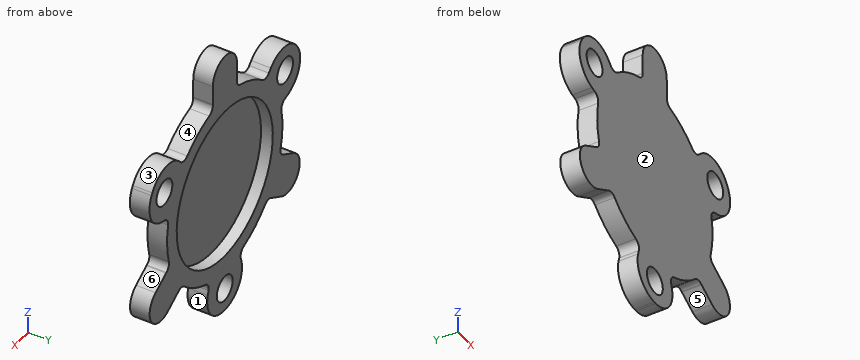
```python
from build123d import *

# Parameters (mm, degrees)
SKETCH1_R           = 20
BOSS_EXTRUDE1_DEPTH = 2
SKETCH2_R           = 35
SKETCH2_R_2         = 20
SKETCH2_R_3         = 3.3
BOSS_EXTRUDE2_DEPTH = 5
CUT_EXTRUDE1_DEPTH  = 10
FILLET1_R           = 2
FILLET2_R           = 7
BOSS_EXTRUDE3_DEPTH = 5
FILLET3_R           = 2


with BuildPart() as part:
    # Sketch1 → Boss-Extrude1 (new body)
    with BuildSketch(Plane(origin=(0, 0, 0), x_dir=(1, 0, 0), z_dir=(0, 1, 0))):
        with Locations(Location((0, 0, 0), (0, 0, 270))):
            Circle(SKETCH1_R)
    extrude(amount=BOSS_EXTRUDE1_DEPTH)

    # Sketch2 → Boss-Extrude2 (add)
    with BuildSketch(Plane(origin=(0, 0, 0), x_dir=(1, 0, 0), z_dir=(0, 1, 0))):
        with Locations(Location((0, 0, 0), (0, 0, 270))):
            Circle(SKETCH2_R)
        with Locations(Location((0, 0, 0), (0, 0, 270))):
            Circle(SKETCH2_R_2, mode=Mode.SUBTRACT)
        with Locations(Location((0, 29, 0), (0, 0, 270))):
            Circle(SKETCH2_R_3, mode=Mode.SUBTRACT)
        with Locations(Location((25.11473671, -14.5, 0), (0, 0, 270))):
            Circle(SKETCH2_R_3, mode=Mode.SUBTRACT)
        with Locations(Location((-25.11473671, -14.5, 0), (0, 0, 270))):
            Circle(SKETCH2_R_3, mode=Mode.SUBTRACT)
    extrude(amount=BOSS_EXTRUDE2_DEPTH)

    # Sketch3 → Cut-Extrude1 (cut)
    with BuildSketch(Plane(origin=(0, 5, 0), x_dir=(1, 0, 0), z_dir=(0, 1, 0))):
        with BuildLine():
            ThreePointArc((-23.193270109, -6.170269172), (-20.763157745, 12.037079399), (-6.170269172, 23.193270109))
            Line((-6.170269172, 23.193270109), (-14.951119735, 56.199389167))
            Line((-14.951119735, 56.199389167), (-49.377364183, -13.136208329))
            Line((-49.377364183, -13.136208329), (-23.193270109, -6.170269172))
        make_face()
        with BuildLine():
            Line((13.312391969, 49.330155919), (6.253025204, 23.171095697))
            ThreePointArc((6.253025204, 23.171095697), (20.805995419, 11.96288237), (23.171095697, -6.253025204))
            Line((23.171095697, -6.253025204), (56.145658563, -15.151645078))
            Line((56.145658563, -15.151645078), (13.312391969, 49.330155919))
        make_face()
        with BuildLine():
            Line((36.064972214, -36.193947589), (16.940244905, -17.000826525))
            ThreePointArc((16.940244905, -17.000826525), (-0.042837674, -23.999961769), (-17.000826525, -16.940244905))
            Line((-17.000826525, -16.940244905), (-41.194538828, -41.047744089))
            Line((-41.194538828, -41.047744089), (36.064972214, -36.193947589))
        make_face()
    extrude(amount=-CUT_EXTRUDE1_DEPTH, mode=Mode.SUBTRACT)

    # Fillet1
    fillet1_edges = [part.edges().sort_by_distance(p)[0] for p in [
        (16.940244905, 2.5, 17.000826525),
        (-17.000826525, 2.5, 16.940244905),
        (6.253025204, 2.5, -23.171095697),
        (23.171095697, 2.5, 6.253025204),
        (-6.170269172, 2.5, -23.193270109),
        (-23.193270109, 2.5, 6.170269172),
    ]]
    fillet(fillet1_edges, radius=FILLET1_R)

    # Fillet2
    fillet2_edges = [part.edges().sort_by_distance(p)[0] for p in [
        (-24.792872016, 2.5, 24.70452382),
        (24.70452382, 2.5, 24.792872016),
        (33.791181225, 2.5, 9.118995089),
        (9.118995089, 2.5, -33.791181225),
        (-8.998309209, 2.5, -33.823518909),
        (-33.823518909, 2.5, 8.998309209),
    ]]
    fillet(fillet2_edges, radius=FILLET2_R)

    # Sketch4 → Boss-Extrude3 (add)
    with BuildSketch(Plane(origin=(0, 5, 0), x_dir=(1, 0, 0), z_dir=(0, 1, 0))):
        with BuildLine():
            Line((-23.70496499, 19.52200868), (-19.379307126, 17.014283806))
            ThreePointArc((-19.379307126, 17.014283806), (-17.561374138, 10.180901067), (-24.394756876, 8.362968079))
            Line((-24.394756876, 8.362968079), (-28.720414739, 10.870692953))
            ThreePointArc((-28.720414739, 10.870692953), (-30.538347728, 17.704075692), (-23.70496499, 19.52200868))
        make_face()
        with BuildLine():
            Line((23.774503624, 19.437262295), (19.439921245, 16.944995134))
            ThreePointArc((19.439921245, 16.944995134), (17.597606027, 10.118145595), (24.424455566, 8.275830376))
            Line((24.424455566, 8.275830376), (28.759037945, 10.768097537))
            ThreePointArc((28.759037945, 10.768097537), (30.601353164, 17.594947076), (23.774503624, 19.437262295))
        make_face()
        with BuildLine():
            Line((4.945911115, -30.307955248), (4.954835631, -25.307963213))
            ThreePointArc((4.954835631, -25.307963213), (-0.036231889, -20.299046662), (-5.04514844, -25.290114182))
            Line((-5.04514844, -25.290114182), (-5.054072955, -30.290106217))
            ThreePointArc((-5.054072955, -30.290106217), (-0.063005435, -35.299022768), (4.945911115, -30.307955248))
        make_face()
    extrude(amount=-BOSS_EXTRUDE3_DEPTH)

    # Fillet3
    fillet3_edges = [part.edges().sort_by_distance(p)[0] for p in [
        (-18.017295098, 2.5, -15.854875507),
        (-22.711825842, 2.5, -7.757123623),
        (22.739372512, 2.5, -7.675997509),
        (18.073779039, 2.5, -15.790456334),
        (-4.722077413, 2.5, 23.530873016),
        (4.638046803, 2.5, 23.547579957),
    ]]
    fillet(fillet3_edges, radius=FILLET3_R)


solid = part.part
```
Build history of the part. All positions in model axes, mm. Face numbers are marked on the shaded views. A direction names the side the tool comes from. Round coordinates to 2 decimals unless told otherwise and drop trailing zeros. Write each loop counter-clockwise with the first axis right and the second up, starting at its lowest first coordinate (ties: lowest second). Pieces come first, ordered by that corner, then holes. Notation, with made-up numbers: (33.5, 31) - (73.5, 31) arc R24 cw to (73.5, 42) - close; hole circle Ø6 at (4.5, -29.75). An arc over 180 degrees is marked (long way). Answer as CSV lines item,"result".
Q1. Cut at D-D (y = 1.05). State how many separate pieces and enclosed holes the cut face has, and give its area (3 significant figures).
Report:
separate pieces,"1"
enclosed holes,"3"
area,"2,440 mm^2"
Q2. Pull direction X, two halves, no side cores. Call the marked faces 1, 2 and 3: +X half, -X half, draft (parallel to the pull), parting line (faces both ways), or undercut.
Report:
face 1,"+X half"
face 2,"draft"
face 3,"undercut"
Q3. Tool access for the marked faces 4, 5 and 6: list every direction of +Z, -Z, +X, -X, +Y, -Y with a clear straight run to the whole face (end or side of a thin tool).
Report:
face 4,"+Z, +Y, -Y"
face 5,"-Z, +Y, -Y"
face 6,"+X, +Y, -Y"
Q4. Cut at A-A (z = 14.5). Write the cut outline in (x, y).
Report:
outline,"(-31.36, 0) - (-28.41, 0) - (-28.41, 5) - (-31.36, 5) - close; (-21.81, 0) - (21.81, 0) - (21.81, 5) - (13.77, 5) - (13.77, 2) - (-13.77, 2) - (-13.77, 5) - (-21.81, 5) - close; (28.41, 0) - (31.32, 0) - (31.32, 5) - (28.41, 5) - close"
Q5. Drill centre lines: probe 1 along Z at (x, y) = (-26, 3.2); probe 2 along X at (y, z) = (3.55, 12.5); probe 3 along X at (y, z) = (1.8, 14.5). Where is each one in solid material? Low to high. Write a range as [from, to].
Report:
probe 1,"z = [-20.19, -9.29], [6.92, 11.32], [17.68, 20.93]"
probe 2,"x = [-31.29, -27.74], [-22.49, -15.61], [15.61, 22.49], [27.74, 31.22]"
probe 3,"x = [-31.36, -28.41], [-21.81, 21.81], [28.41, 31.32]"
Q6. Cut at C-C (z = -29). Write the cut outline in (x, y), and give its area (3 significant figures).
Report:
outline,"(-7.13, 0) - (-3.3, 0) - (-3.3, 5) - (-7.13, 5) - close; (3.3, 0) - (7.23, 0) - (7.23, 5) - (3.3, 5) - close"
area,"38.8 mm^2"
Q7. Drop flat-ended pins along their axis: pin 1 (6 mm diameter, centred on x = 13, z = -24, fed in from +Y); pin 2 (2 mm diameter, centred on x = 20.5, y = 0.5, fed in from -Z); pin 3 (12 mm diameter, centred on x = -8.5, z = -9.5, fed in from +Y). Give the stop position or say it passes through.
Report:
pin 1,"passes through"
pin 2,"stops at z = -18.13"
pin 3,"stops at y = 2"
Q8. Cut at B-B (z = 0). Write the cut outline in (x, y).
Report:
outline,"(-24, 0) - (24, 0) - (24, 5) - (20, 5) - (20, 2) - (-20, 2) - (-20, 5) - (-24, 5) - close"
